```python
from build123d import *

# Parameters (mm, degrees)
SKETCH1_W           = 137
SKETCH1_H           = 72
BOSS_EXTRUDE1_DEPTH = 16
SKETCH2_W           = 5
SKETCH2_H           = 12.5
CUT_EXTRUDE1_DEPTH  = 12
FILLET1_R           = 10
FILLET2_R           = 3
FILLET3_R           = 3


with BuildPart() as part:
    # Sketch1 → Boss-Extrude1 (new body)
    with BuildSketch(Plane.XY):
        with Locations((-68.5, 36)):
            Rectangle(SKETCH1_W, SKETCH1_H)
    extrude(amount=BOSS_EXTRUDE1_DEPTH)

    # Sketch2 → Cut-Extrude1 (cut)
    with BuildSketch(Plane.ZY.offset(137)):
        with Locations((8, 52.75)):
            Rectangle(SKETCH2_W, SKETCH2_H)
        with Locations((8, 19.25)):
            Rectangle(SKETCH2_W, SKETCH2_H)
    extrude(amount=-CUT_EXTRUDE1_DEPTH, mode=Mode.SUBTRACT)

    # Fillet1
    fillet1_edges = [part.edges().sort_by_distance(p)[0] for p in [
        (0, 0, 8),
        (-137, 0, 8),
        (-137, 72, 8),
        (0, 72, 8),
    ]]
    fillet(fillet1_edges, radius=FILLET1_R)

    # Fillet2
    fillet2_edges = [part.edges().sort_by_distance(p)[0] for p in [
        (-68.5, 0, 0),
        (0, 36, 0),
        (-137, 36, 0),
        (-68.5, 72, 0),
        (-134.071067812, 69.071067812, 0),
        (-2.928932188, 69.071067812, 0),
        (-2.928932188, 2.928932188, 0),
        (-134.071067812, 2.928932188, 0),
    ]]
    fillet(fillet2_edges, radius=FILLET2_R)

    # Fillet3
    fillet3_edges = [part.edges().sort_by_distance(p)[0] for p in [
        (-68.5, 0, 16),
        (-137, 36, 16),
        (0, 36, 16),
        (-68.5, 72, 16),
        (-134.071067812, 69.071067812, 16),
        (-2.928932188, 69.071067812, 16),
        (-2.928932188, 2.928932188, 16),
        (-134.071067812, 2.928932188, 16),
    ]]
    fillet(fillet3_edges, radius=FILLET3_R)


solid = part.part
```
Geometry check sheet. Reference: the model listing, model coordinates, mm. A direction names the side the tool comes from. Round coordinates to 2 decimals unless told otherwise and drop trailing zeros. Order: outer loops, then holes, each group sorted by start corner. A loop starts at its lowest first (then second) coordinate and runs counter-clockwise, first axis right, second up. Notation, with made-up numbers: (19, -12.75) - (77, -12.75) arc R36 cw to (77, 22.25) - close; hole circle Ø9 at (60, 85). An arc over 180 degrees is marked (long way). Use a Markdown table: item, result. Add a question column.
1) Section check B-B (y = 21.5). Record the cut outline in (x, z), then the cut area to 3 significant figures.
2) Mould release check, pull along Y, two halves, no side actions. Record for faces 3 (the flat face through (-131, 19, 10.5)), 4 (the cylindrical face through (-136.1, 35.64, 15.14)), 5 (the cylindrical face through (-3.01, 2.85, 8.07)): released by +Y, released by -Y, zero draft, split by the parting line, or undercut.
3) Set-up check for faces 1 (the flat face through (-137, 36, 8)), 2 (the flat face through (-131, 53, 5.5)): record each of +Z, -Z, +X, -X, +Y, -Y from which the full face is reachable in a straight line by a thin tool's end or side.
4) Thickness scan on line 1 along Z through (x, y) = (-130, 58); line 2 along X through (y, z) = (16.5, 6.25); line 3 along Y through (x, z) = (-9.5, 11.75). Record the ranges inside material, lowest first.
5) Section check C-C (z = 14.5). Record the cut outline in (x, y), then the cut area to 3 significant figures.
6) Section check A-A (z = 7). Record the cut outline in (x, y), then the cut area to 3 significant figures.
7) Gauge pin test, flat ends, axial feed: P1, Ø2, axis at x = -82.5, z = 13.5, coming from the -Y side; P2, Ø5.5, axis at x = -132.5, z = 8, coming from the -Y side; P3, Ø2.5, axis at x = -130, z = 7.5, coming from the +Y side; P4, Ø1.5, axis at y = 20.5, z = 1.5, coming from the +X side. Record the tip position at first contact, or that the pin passes through.
Established:
| question | item | result |
|---|---|---|
| 1 | outline | (-137, 3) arc R3 ccw to (-134, 0) - (-3, 0) arc R3 ccw to (0, 3) - (0, 13) arc R3 ccw to (-3, 16) - (-134, 16) arc R3 ccw to (-137, 13) - (-137, 10.5) - (-125, 10.5) - (-125, 5.5) - (-137, 5.5) - close |
| 1 | area | 2,120 mm2 |
| 2 | face 3 | undercut |
| 2 | face 4 | zero draft |
| 2 | face 5 | released by -Y |
| 3 | face 1 | +Z, -Z, -X, +Y, -Y |
| 3 | face 2 | -X |
| 4 | line 1 | 0 to 5.5, 10.5 to 16 |
| 4 | line 2 | -125 to 0 |
| 4 | line 3 | 0.01 to 71.99 |
| 5 | outline | (-136.6, 10) arc R9.6 ccw to (-127, 0.4) - (-10, 0.4) arc R9.6 ccw to (-0.4, 10) - (-0.4, 62) arc R9.6 ccw to (-10, 71.6) - (-127, 71.6) arc R9.6 ccw to (-136.6, 62) - close |
| 5 | area | 9,620 mm2 |
| 6 | outline | (-137, 10) arc R10 ccw to (-127, 0) - (-10, 0) arc R10 ccw to (0, 10) - (0, 62) arc R10 ccw to (-10, 72) - (-127, 72) arc R10 ccw to (-137, 62) - (-137, 59) - (-125, 59) - (-125, 46.5) - (-137, 46.5) - (-137, 25.5) - (-125, 25.5) - (-125, 13) - (-137, 13) - close |
| 6 | area | 9,480 mm2 |
| 7 | P1 | y = 0 |
| 7 | P2 | y = 0.39 |
| 7 | P3 | y = 71.85 |
| 7 | P4 | x = -0.1 |
